```python
from build123d import *

# Parameters (mm, degrees)
BOSS_EXTRUDE2_DEPTH        = 3
SKETCH5_R                  = 1.5
CUT_EXTRUDE3_DEPTH         = 3
SKETCHED_START             = 72.251106428
SKETCHED_BEND2_OUTLINE_W   = 3
SKETCHED_BEND2_OUTLINE_H   = 15
SKETCHED_BEND2_DEPTH       = 85.748893572
SKETCHED_START_2           = 69.251106428
SKETCHED_BEND2_2_OUTLINE_R = 1.5
SKETCHED_BEND2_2_DEPTH     = 2.5137
SKETCHED_START_3           = 67.251106428
SKETCHED_BEND2_3_OUTLINE_R = 1.5
SKETCHED_BEND2_3_DEPTH     = 5
SKETCHED_START_4           = -107
SKETCHED_BEND2_4_DEPTH     = 17
SKETCHED_START_5           = -105.530592626
SKETCHED_BEND3_DEPTH       = 15
SKETCHED_BEND3_2_DEPTH     = 15
SKETCH26_W                 = 8
SKETCH26_H                 = 2.5
CUT_EXTRUDE8_DEPTH         = 10


with BuildPart() as part:
    # Sketch1 → Boss-Extrude2 (new body)
    with BuildSketch(Plane(origin=(0, 0, 0), x_dir=(1, 0, 0), z_dir=(0, 1, 0))):
        with BuildLine():
            Line((150, 105.530592626), (0, 105.530592626))
            Line((0, 105.530592626), (0, 90.530592626))
            Line((0, 90.530592626), (103.25004789, 90.530592626))
            Line((103.25004789, 90.530592626), (150, 90.530592626))
            ThreePointArc((150, 90.530592626), (157.5, 98.030592626), (150, 105.530592626))
        make_face()
    extrude(amount=BOSS_EXTRUDE2_DEPTH)

    # Sketch5 → Cut-Extrude3 (cut)
    with BuildSketch(Plane(origin=(0, 3, 0), x_dir=(1, 0, 0), z_dir=(0, 1, 0))):
        with Locations(Location((135, 98.030592626, 0), (0, 0, 270))):
            Circle(SKETCH5_R)
    extrude(amount=-CUT_EXTRUDE3_DEPTH, mode=Mode.SUBTRACT)

    # Sketched Bend2: read off the stored shape, not the designer's step
    # Sketched Bend2 outline → Sketched Bend2 (cut)
    with BuildSketch(Plane.YZ.offset(SKETCHED_START)):
        with Locations((1.5, -98.030592626)):
            Rectangle(SKETCHED_BEND2_OUTLINE_W, SKETCHED_BEND2_OUTLINE_H)
    extrude(amount=SKETCHED_BEND2_DEPTH, mode=Mode.SUBTRACT)

    # Sketched Bend2 2 outline → Sketched Bend2 2 (add)
    with BuildSketch(Plane.YZ.offset(SKETCHED_START_2)):
        with BuildLine():
            Line((0, -90.530592626), (-79.251106428, -90.530592626))
            ThreePointArc((-79.251106428, -90.530592626), (-86.751106428, -98.030592626), (-79.251106428, -105.530592626))
            Line((-79.251106428, -105.530592626), (0, -105.530592626))
            Line((0, -105.530592626), (0, -90.530592626))
        make_face()
        with Locations((-64.251106428, -98.030592626)):
            Circle(SKETCHED_BEND2_2_OUTLINE_R, mode=Mode.SUBTRACT)
    extrude(amount=SKETCHED_BEND2_2_DEPTH)

    # Sketched Bend2 3 outline → Sketched Bend2 3 (add)
    with BuildSketch(Plane.YZ.offset(SKETCHED_START_3)):
        with BuildLine():
            Line((0, -90.530592626), (-79.251106428, -90.530592626))
            ThreePointArc((-79.251106428, -90.530592626), (-86.751106428, -98.030592626), (-79.251106428, -105.530592626))
            Line((-79.251106428, -105.530592626), (0, -105.530592626))
            Line((0, -105.530592626), (0, -90.530592626))
        make_face()
        with Locations((-64.251106428, -98.030592626)):
            Circle(SKETCHED_BEND2_3_OUTLINE_R, mode=Mode.SUBTRACT)
    extrude(amount=SKETCHED_BEND2_3_DEPTH)

    # Sketched Bend2 4 outline → Sketched Bend2 4 (cut)
    with BuildSketch(Plane.XY.offset(SKETCHED_START_4)):
        with BuildLine():
            Line((69.251106428, -88), (69.251106428, -2))
            ThreePointArc((69.251106428, -2), (68.66531999, -0.585786438), (67.251106428, 0))
            Line((67.251106428, 0), (67.251106428, -88))
            Line((67.251106428, -88), (69.251106428, -88))
        make_face()
        with BuildLine():
            Line((72.251106428, -2), (72.251106424, -88))
            Line((72.251106424, -88), (74, -88))
            Line((74, -88), (74, 4))
            Line((74, 4), (66, 4))
            Line((66, 4), (66, 3))
            Line((66, 3), (67.251106428, 3))
            ThreePointArc((67.251106428, 3), (70.786640334, 1.535533906), (72.251106428, -2))
        make_face()
    extrude(amount=SKETCHED_BEND2_4_DEPTH, mode=Mode.SUBTRACT)

    # Sketched Bend3: read off the stored shape, not the designer's step
    # Sketched Bend3 outline → Sketched Bend3 (cut)
    with BuildSketch(Plane.XY.offset(SKETCHED_START_5)):
        with BuildLine():
            ThreePointArc((45, 0), (42.261387212, 0.816699867), (40.417424305, 3))
            Line((40.417424305, 3), (0, 3))
            Line((0, 3), (0, 0))
            Line((0, 0), (45, 0))
        make_face()
    extrude(amount=SKETCHED_BEND3_DEPTH, mode=Mode.SUBTRACT)

    # Sketched Bend3 2 outline → Sketched Bend3 2 (add)
    with BuildSketch(Plane.XY.offset(SKETCHED_START_5)):
        with BuildLine():
            ThreePointArc((45, 3), (43.585786438, 3.585786438), (43, 5))
            Line((43, 5), (43, 44.502212856))
            Line((43, 44.502212856), (40, 44.502212856))
            Line((40, 44.502212856), (40, 5))
            ThreePointArc((40, 5), (40.105468435, 3.978451782), (40.417424305, 3))
            Line((40.417424305, 3), (45, 3))
        make_face()
    extrude(amount=SKETCHED_BEND3_2_DEPTH)

    # Sketch26 → Cut-Extrude8 (cut)
    with BuildSketch(Plane(origin=(43, 0, 0), x_dir=(0, 0, -1), z_dir=(1, 0, 0))):
        with Locations((96.530592626, 43.252212856)):
            Rectangle(SKETCH26_W, SKETCH26_H)
    extrude(amount=-CUT_EXTRUDE8_DEPTH, mode=Mode.SUBTRACT)


solid = part.part
```
For this review, take the finished solid that the model builds, in its own axes (mm). A direction names the side the tool comes from. Round coordinates to 2 decimals unless told otherwise and drop trailing zeros. Order: outer loops, then holes, each group sorted by start corner. A loop starts at its lowest first (then second) coordinate and runs counter-clockwise, first axis right, second up.
Q1. Mouldability with a two-part tool opening along Z and no side actions: class faces 6 (the flat face through (69.251, -45, -98)), 7 (the flat face through (57, 1, -105.531)), 8 (the cylindrical face through (70.73, -86.75, -97.87)), 9 (the flat face through (42, 42.002, -96)) as pulls with the +Z half, pulls with the -Z half, needs draft (parallel to the pull), parting line crosses it, or undercut.
Findings below:
face 6: needs draft
face 7: pulls with the -Z half
face 8: parting line crosses it
face 9: undercut
Q2. We need section A-A, the plane y = 12.5. Give the boundary of the cut face in (x, z).
Findings below:
outline: (40, -105.53) - (43, -105.53) - (43, -90.53) - (40, -90.53) - close
Q3. Insertion check: P1, Ø3, axis at y = -25.5, z = -103.5, coming from the -X side; P2, Ø2.5, axis at y = -64.25, z = -98.03, coming from the +X side; P3, Ø3, axis at x = 45, z = -94, coming from the +Y side; P4, Ø1.5, axis at x = 41, z = -96.5, coming from the +Y side. Each pin has a flat end and moves straight along its axis. Give the tip position at first contact, or say it passes through.
Findings below:
P1: stops at x = 69.25
P2: passes through
P3: stops at y = 3.68
P4: stops at y = 42
Q4. Wall thickness on line 1 (X direction, y = -76.5, z = -104); line 2 (X direction, y = 19, z = -98.5); line 3 (Y direction, x = 46.5, z = -97.5): over which ranges is each line inside the solid? List them lowest first.
Findings below:
line 1: x = 69.25 to 72.25
line 2: x = 40 to 43
line 3: y = 0 to 3
Q5. We need section C-C, the plane z = -102.25. Give the boundary of the cut face in (x, y), plus the area to 3 significant figures.
Findings below:
outline: (40, 5) arc R5 ccw to (45, 0) - (67.25, 0) arc R2 cw to (69.25, -2) - (69.25, -85.45) - (72.25, -85.45) - (72.25, -2) arc R5 ccw to (67.25, 3) - (45, 3) arc R2 cw to (43, 5) - (43, 44.5) - (40, 44.5) - close
area: 469 mm2
Q6. Machinability: for faces 1 (the flat face through (56, 3, -98)), 2 (the flat face through (57, 1, -90.531)), 3 (the cylindrical face through (70.73, -65.441, -98.943)), 4 (the flat face through (42, 43, -92.531)), 5 (the flat face through (56, 0, -98)), which of the approach directions +Z, -Z, +X, -X, +Y, -Y give a long, thin tool a straight path to every point of the face, cutting with its end or side? Answer none if there is none.
Findings below:
face 1: +Z, -Z, +X, +Y
face 2: +Z, +X, -X, +Y, -Y
face 3: +X, -X
face 4: +X, -X, +Y
face 5: +Z, -Z, -X, -Y
Q7. We need section B-B, the plane x = 59. Give the boundary of the cut face in (y, z).
Findings below:
outline: (0, -105.53) - (3, -105.53) - (3, -90.53) - (0, -90.53) - close
